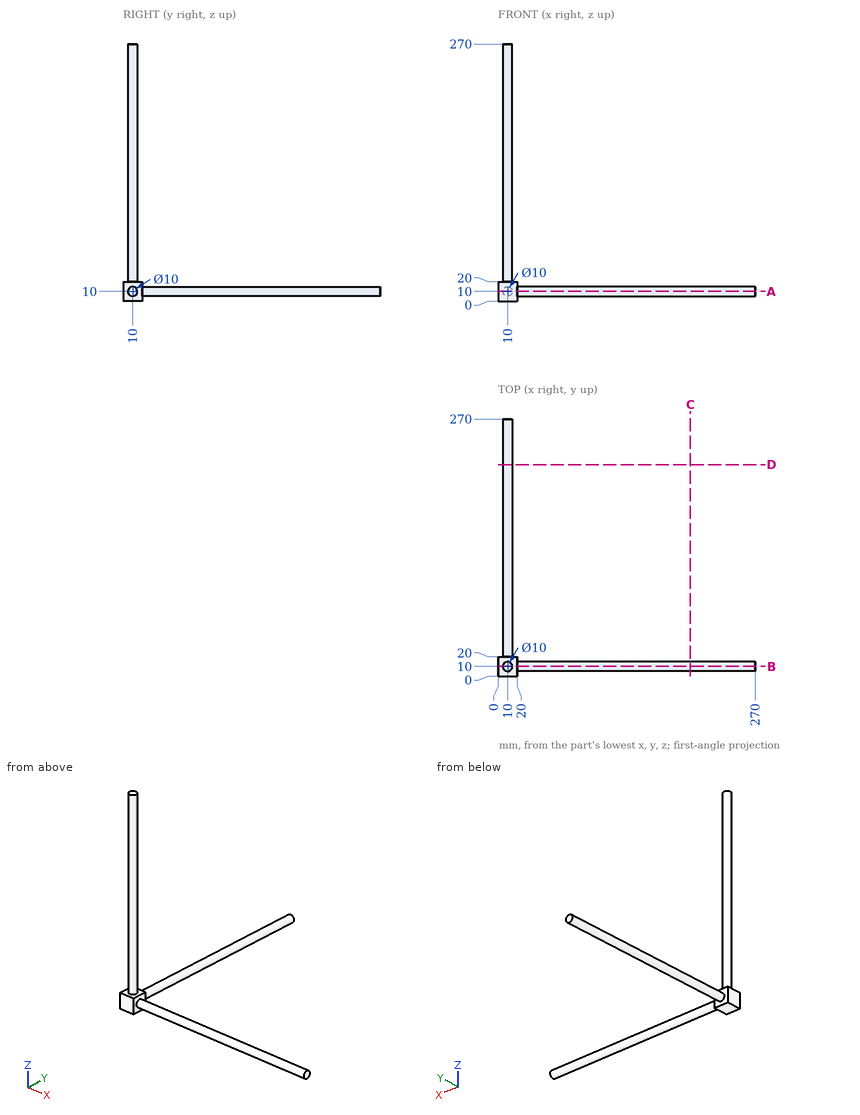
Here's the drawing with two shaded views (mm, measured from the low corner). I have some questions. Round coordinates to 2 decimals unless told otherwise and drop trailing zeros. Loops run counter-clockwise (first coordinate to the right, second up) from the corner with the lowest first, then second, coordinate; pieces in that order, holes last.
1. If I drill on probe 1 along Z at (x, y) = (12.5, 76.5); probe 2 along Z at (x, y) = (200, 12), over which ranges is the centre line in solid material (lowest first)?
Answers:
probe 1: z = 5.67 to 14.33
probe 2: z = 5.42 to 14.58
2. Suppose I cut it at C-C, the plane x = 202. Please give me the cut outline in (y, z), and give its area (3 significant figures).
Answers:
outline: circle Ø10 at (10, 10)
area: 78.5 mm2
3. Suppose I cut it at A-A, the plane z = 10. Please give me the cut outline in (x, y), and give its area (3 significant figures).
Answers:
outline: (0, 0) - (20, 0) - (20, 5) - (270, 5) - (270, 15) - (20, 15) - (20, 20) - (15, 20) - (15, 270) - (5, 270) - (5, 20) - (0, 20) - close
area: 5,400 mm2
